Could you check a few things on this model? Use its own coordinates, in mm. Face numbers are marked on the shaded views. Round coordinates to 2 decimals unless told otherwise and drop trailing zeros. Loops run counter-clockwise (first coordinate to the right, second up) from the corner with the lowest first, then second, coordinate; pieces in that order, holes last.
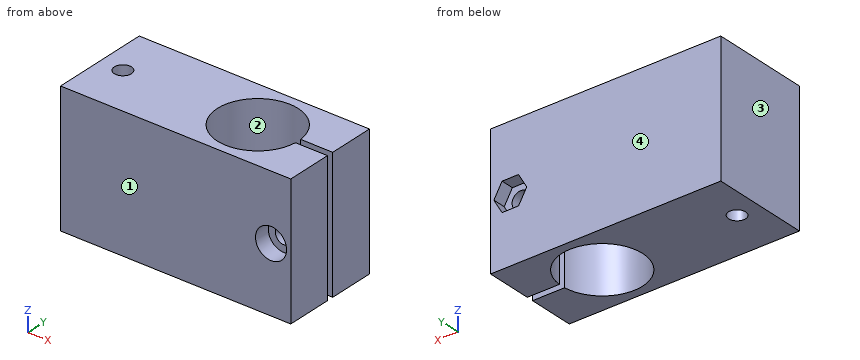
from build123d import *

# Parameters (mm, degrees)
F0_R     = 1.65
F1_DEPTH = 12.7
F2_R     = 1.65
F3_DEPTH = 25.4
F4_R     = 3
F4_R_2   = 1.65
F5_DEPTH = 3.1
F6_R     = 1.65
F7_DEPTH = 2.5


with BuildPart() as f1:
    # F0 (on Top) → F1 (new body, symmetric)
    with BuildSketch(Plane.XY):
        with BuildLine():
            Line((22.225, 9.525), (-22.225, 9.525))
            Line((-22.225, 9.525), (-22.225, -9.525))
            Line((-22.225, -9.525), (22.225, -9.525))
            Line((22.225, -9.525), (22.225, -0.635))
            Line((22.225, -0.635), (16.039644, -0.635))
            ThreePointArc((16.039644, -0.635), (0.4445, 0), (16.039644, 0.635))
            Line((16.039644, 0.635), (22.225, 0.635))
            Line((22.225, 0.635), (22.225, 9.525))
        make_face()
        with Locations((-17.78, 0)):
            Circle(F0_R, mode=Mode.SUBTRACT)
    extrude(amount=F1_DEPTH, both=True)

    # F2 (on Front) → F3 (cut, symmetric)
    with BuildSketch(Plane.XZ):
        with Locations((18.415, 0)):
            Circle(F2_R)
    extrude(amount=F3_DEPTH, both=True, mode=Mode.SUBTRACT)

    # F4 (on face) → F5 (cut)
    with BuildSketch(Plane.XZ.offset(9.525)):
        with Locations((18.415, 0)):
            Circle(F4_R)
        with Locations((18.415, 0)):
            Circle(F4_R_2, mode=Mode.SUBTRACT)
    extrude(amount=-F5_DEPTH, mode=Mode.SUBTRACT)

    # F6 (on face) → F7 (cut)
    with BuildSketch(Plane(origin=(0, 9.525, 0), x_dir=(-1, 0, 0), z_dir=(0, 1, 0))):
        Polygon((-16.827287, 2.75), (-20.002713, 2.75), (-21.590426, 0), (-20.002713, -2.75), (-16.827287, -2.75), (-15.239574, 0), align=None)
        with Locations((-18.415, 0)):
            Circle(F6_R, mode=Mode.SUBTRACT)
    extrude(amount=-F7_DEPTH, mode=Mode.SUBTRACT)


solid = f1.part
Item 1: If we section it at A-A, the plane x = -17.78: Please give me the cut outline in (y, z) (3 decimals).
Results list:
outline: (-9.525, -12.7) - (-1.65, -12.7) - (-1.65, 12.7) - (-9.525, 12.7) - close; (1.65, -12.7) - (9.525, -12.7) - (9.525, 12.7) - (1.65, 12.7) - close
Item 2: Will these pins go through, and if not, where does the flat tip stop? pin 1 (3.5 mm diameter, centred on x = 18.415, z = 0, fed in from -Y) (3 decimals); pin 2 (2.5 mm diameter, centred on x = 18.415, z = 0, fed in from +Y).
Results list:
pin 1: stops at y = -6.425
pin 2: passes through
Item 3: If we section it at C-C, the plane y = -2.25: Please give me the cut outline in (x, z) (3 decimals), then the cut area to 3 significant figures.
Results list:
outline: (-22.225, -12.7) - (0.776, -12.7) - (0.776, 12.7) - (-22.225, 12.7) - close; (15.734, -12.7) - (22.225, -12.7) - (22.225, 12.7) - (15.734, 12.7) - close; hole circle Ø3.3 at (18.415, 0)
area: 741 mm2
Item 4: If we section it at D-D, the plane y = 0: Please give me the cut outline in (x, z) (1 decimal), then the cut area to 3 significant figures.
Results list:
outline: (-22.2, -12.7) - (-19.4, -12.7) - (-19.4, 12.7) - (-22.2, 12.7) - close; (-16.1, -12.7) - (0.4, -12.7) - (0.4, 12.7) - (-16.1, 12.7) - close
area: 492 mm2
Item 5: If I drill on line 1 along Y through (x, z) = (-17.78, -5.25) (3 decimals); line 2 along Z through (x, y) = (18.5, -4.25); line 3 along Y through (x, z) = (17.5, -5) (3 decimals), over which ranges is the centre line in solid material (lowest first)?
Results list:
line 1: y = -9.525 to -1.65, 1.65 to 9.525
line 2: z = -12.7 to -1.65, 1.65 to 12.7
line 3: y = -9.525 to -0.635, 0.635 to 9.525
Item 6: We'd pull the mould along Y, two halves only. Please class the marked faces 1, 2, 3 and 4: released by +Y, released by -Y, zero draft, split by the parting line, or undercut.
Results list:
face 1: released by -Y
face 2: undercut
face 3: zero draft
face 4: released by +Y
